```python
from build123d import *

# Parameters (mm, degrees)
EXTRUDE_1_DEPTH        = 700
EXTRUDE_1_2_DEPTH      = 20
EXTRUDE_1_2_DEPTH_BACK = 20
SKETCH_2_R             = 30
EXTRUDE_START          = 20
SKETCH_3_R             = 30
SKETCH_3_W             = 25
SKETCH_3_H             = 25
EXTRUDE_2_DEPTH        = 20
CUT_EXTRUDE_1_DEPTH    = 742.531523268
PATTERN_LINEAR_1_COUNT = 13
PATTERN_LINEAR_1_PITCH = 30
CUT_EXTRUDE_2_DEPTH    = 742.531523268
PATTERN_LINEAR_2_COUNT = 13
PATTERN_LINEAR_2_PITCH = 30
CUT_EXTRUDE_3_DEPTH    = 5
SKETCH_11_OUTSIDE_W    = 209.976
SKETCH_11_OUTSIDE_H    = 209.976
SKETCH_11_OUTSIDE_R    = 30
CUT_EXTRUDE_4_DEPTH    = 735


with BuildPart() as part:
    # 草图1 → Extrude 1 (new body)
    with BuildSketch(Plane(origin=(0, 0, 0), x_dir=(1, 0, 0), z_dir=(0, 1, 0))):
        Polygon((30, 0), (0, 0), (0, -30), (7, -30), (7, -7), (30, -7), align=None)
    extrude(amount=EXTRUDE_1_DEPTH)

    # 草图2 → Extrude 1 2 (add, two sides: drawn at the far end of the back side and taken through both)
    with BuildSketch(Plane(origin=(0, 700, 0), x_dir=(1, 0, 0), z_dir=(0, 1, 0)).offset(-EXTRUDE_1_2_DEPTH_BACK)):
        with Locations(Location((0, 0, 0), (0, 0, 270))):
            Circle(SKETCH_2_R)
    extrude(amount=EXTRUDE_1_2_DEPTH + EXTRUDE_1_2_DEPTH_BACK)

    # 草图3 → 凸台-拉伸2 (add)
    with BuildSketch(Plane(origin=(0, 720, 0), x_dir=(1, 0, 0), z_dir=(0, 1, 0)).offset(EXTRUDE_START)):
        with Locations(Location((0, 0, 0), (0, 0, 270))):
            Circle(SKETCH_3_R)
        Rectangle(SKETCH_3_W, SKETCH_3_H, mode=Mode.SUBTRACT)
    extrude(amount=-EXTRUDE_2_DEPTH)

    # 草图6 → 切除-拉伸1 (cut, through all)
    with BuildSketch(Plane.XY.offset(7)):
        with BuildLine():
            Line((23.5, 30), (23.5, 20))
            ThreePointArc((23.5, 20), (18.5, 15), (13.5, 20))
            Line((13.5, 20), (13.5, 30))
            ThreePointArc((13.5, 30), (18.5, 35), (23.5, 30))
        make_face()
    cut_extrude_1 = extrude(amount=-CUT_EXTRUDE_1_DEPTH, mode=Mode.SUBTRACT)

    # 阵列(线性)1: 切除-拉伸1 ×13
    with Locations(*[(0, i * PATTERN_LINEAR_1_PITCH, 0) for i in range(1, PATTERN_LINEAR_1_COUNT)]):
        add(cut_extrude_1, mode=Mode.SUBTRACT)

    # 草图7 → 切除-拉伸2 (cut, through all)
    with BuildSketch(Plane(origin=(7, 0, 0), x_dir=(0, 0, -1), z_dir=(1, 0, 0))):
        with BuildLine():
            Line((-23.5, 20), (-23.5, 30))
            ThreePointArc((-23.5, 30), (-18.5, 35), (-13.5, 30))
            Line((-13.5, 30), (-13.5, 20))
            ThreePointArc((-13.5, 20), (-18.5, 15), (-23.5, 20))
        make_face()
    cut_extrude_2 = extrude(amount=-CUT_EXTRUDE_2_DEPTH, mode=Mode.SUBTRACT)

    # 阵列(线性)2: 切除-拉伸2 ×13
    with Locations(*[(0, i * PATTERN_LINEAR_2_PITCH, 0) for i in range(1, PATTERN_LINEAR_2_COUNT)]):
        add(cut_extrude_2, mode=Mode.SUBTRACT)

    # 草图8 → 切除-拉伸3 (cut)
    with BuildSketch(Plane.XZ):
        Polygon((30, 7), (7, 7), (7, 30), (0, 30), (0, 0), (30, 0), align=None)
    extrude(amount=-CUT_EXTRUDE_3_DEPTH, mode=Mode.SUBTRACT)

    # 草图11 outside → 切除-拉伸4 (cut)
    with BuildSketch(Plane(origin=(0, 740, 0), x_dir=(1, 0, 0), z_dir=(0, 1, 0))):
        Rectangle(SKETCH_11_OUTSIDE_W, SKETCH_11_OUTSIDE_H)
        with Locations(Location((0, 0, 0), (0, 0, 270))):
            Circle(SKETCH_11_OUTSIDE_R, mode=Mode.SUBTRACT)
    extrude(amount=-CUT_EXTRUDE_4_DEPTH, mode=Mode.SUBTRACT)


solid = part.part
```
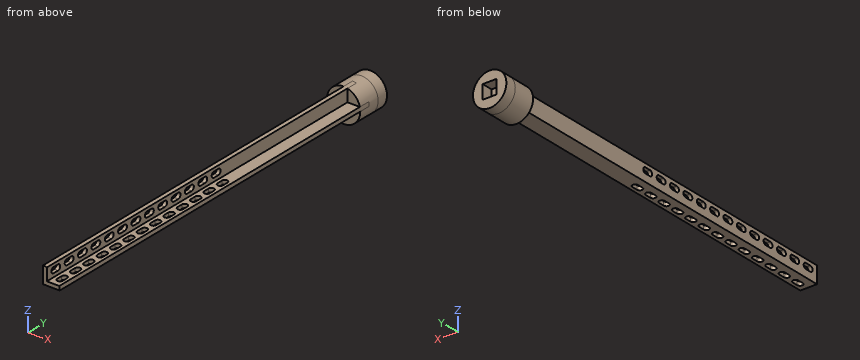
Here's how the part is built. I have some questions about the finished solid (model axes, mm). Round coordinates to 2 decimals unless told otherwise and drop trailing zeros. Order: outer loops, then holes, each group sorted by start corner. A loop starts at its lowest first (then second) coordinate and runs counter-clockwise, first axis right, second up. Notation, with made-up numbers: M 42.25,45 L 62.25,45 A17 ccw 62.25,74 Z; hole C 18,45 d8. An arc over 180 degrees is marked long. Use CSV: the item, a comma, the result in double quotes.
1) I need wall thicknesses on line 1 along Y through (x, z) = (-20.5, -5); line 2 along X through (y, z) = (459, 27). Which ranges of each line are inside material? Lowest first, please. Write a range as [from, to].
Taken from the geometry:
line 1,"[680, 740]"
line 2,"[0, 7]"
2) I want a section at B-B (x = -22.5). List the corners of the cut face in (y, z) for me, then the cut area to 3 significant figures.
Taken from the geometry:
outline,"M 680,-19.84 L 740,-19.84 L 740,19.84 L 680,19.84 Z"
area,"2,380 mm^2"
3) I want a section at A-A (y = 612.5). List the corners of the cut face in (x, z) for me, then the cut area to 3 significant figures.
Taken from the geometry:
outline,"M 0,0 L 30,0 A30 ccw 29.17,7 L 7,7 L 7,29.17 A30 ccw 0,30 Z"
area,"367 mm^2"
4) I'm going to push flat-ended pins straight in: P1, Ø5.5, axis at x = 4, y = 174.5, coming from the +Z side; P2, Ø5.5, axis at x = 3, y = 83, coming from the -Z side; P3, Ø2, axis at x = 5, z = -14, coming from the -Y side; P4, Ø10, axis at x = -8, z = -1, coming from the +Y side. Where does each tip first touch, or does it pass through?
Taken from the geometry:
P1,"z = 29.97"
P2,"z = 0"
P3,"y = 680"
P4,"y = 740"
5) I want a section at C-C (y = 687). List the corners of the cut face in (x, z) for me.
Taken from the geometry:
outline,"C 0,0 d60"
